Study the drawing (mm; zero at the part's minimum x, y, z) and answer. Round coordinates to 2 decimals unless told otherwise and drop trailing zeros. Write each loop counter-clockwise with the first axis right and the second up, starting at its lowest first coordinate (ties: lowest second). Pieces come first, ordered by that corner, then holes. Notation, with made-up numbers: (43.5, 17.5) - (71.5, 17.5) arc R28 cw to (71.5, 40.5) - close; hole circle Ø9 at (-17, 13). An arc over 180 degrees is marked (long way). Use one line per item in the form item = value. Start each with the question number.
1) For a pull along Y with two mould halves and no side action, classify the marked faces 1, 2 and 3 as released by +Y, released by -Y, zero draft, split by the parting line, or undercut.
2) The part is cut by section B-B, the plane z = 2.4. Give the vertices of the cut face in (x, y).
3) Consider line 1 along X through (y, z) = (5.75, 2.1) (1 decimal); line 2 along Y through (x, z) = (6.25, 1.4) (1 decimal); line 3 along X through (y, z) = (5.5, 0.7) (1 decimal). Determine where each line is inside the solid, lowest interval first. Write a range as from..to.
4) The part is cut by section A-A, the plane z = 1.2. Give the vertices of the cut face in (x, y), plus the area to 3 significant figures.
5) Each of these flat-tipped pins is pushed along its axis until it touches: pin 1 (4.5 mm diameter, centred on x = 4.62, y = 4, fed in from +Z); pin 2 (1 mm diameter, centred on y = 2.5, z = 2, fed in from +X). Where does it stop, or does it pass through?
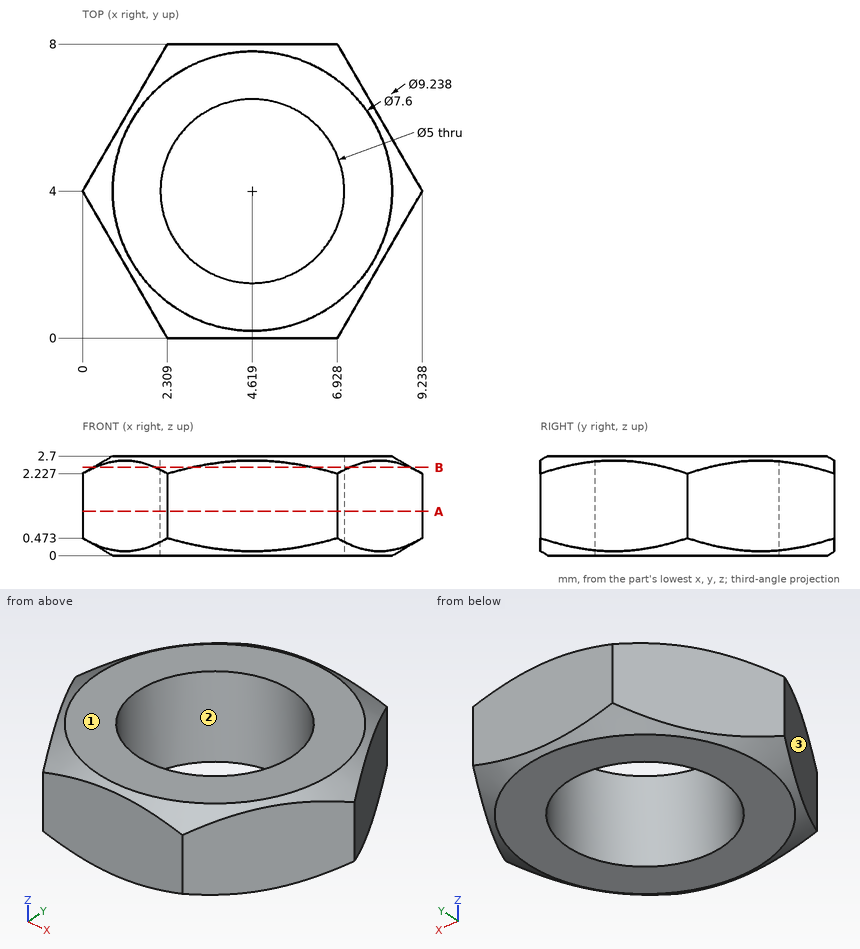
Geometry results:
q1.face_1 = zero draft
q1.face_2 = undercut
q1.face_3 = released by -Y
q2.outline = (0.34, 3.41) - (1.97, 0.59) arc R4.32 ccw to (2.99, 0) - (6.25, 0) arc R4.32 ccw to (7.27, 0.59) - (8.9, 3.41) arc R4.32 ccw to (8.9, 4.59) - (7.27, 7.41) arc R4.32 ccw to (6.25, 8) - (2.99, 8) arc R4.32 ccw to (1.97, 7.41) - (0.34, 4.59) arc R4.32 ccw to start; hole circle Ø5 at (4.62, 4)
q3.line_1 = 1..2.8, 6.4..8.2
q3.line_2 = 0..2.1, 5.9..8
q3.line_3 = 0.9..2.6, 6.6..8.4
q4.outline = (0, 4) - (2.31, 0) - (6.93, 0) - (9.24, 4) - (6.93, 8) - (2.31, 8) - close; hole circle Ø5 at (4.62, 4)
q4.area = 35.8 mm2
q5.pin_1 = through
q5.pin_2 = 8.66
